Can you work these out from the model? Positions are in its coordinate system, mm. A direction names the side the tool comes from. Coordinates: 2 decimals unless noted, no trailing zeros. Loops run counter-clockwise (first coordinate to the right, second up) from the corner with the lowest first, then second, coordinate; pieces in that order, holes last. Notation, with made-up numbers: M 36.5,38.5 L 43.5,38.5 A29 ccw 43.5,67.5 Z; hole C -20.75,-12.5 d7. An arc over 180 degrees is marked long. Answer as a JSON object with one key per item and string values. Group by question number.
Item 1: We'd pull the mould along X, two halves only. Please class faces 3 (the cylindrical face through (16.345, -0.592, -0.479)), 4 (the flat face through (-4.945, -0.592, 35.75)), 5 (the flat face through (8.75, -0.59, -3.48)): +X half, -X half, draft (parallel to the pull), parting line (faces both ways), or undercut.
Item 2: Which directions (+Z, -Z, +X, -X, +Y, -Y) give clear straight access to the entire face, cutting with the end or side of a thin tool? Please do faces 1 (the flat face through (12.65, -0.59, 3.34)), 2 (the flat face through (5.34, -0.59, 15.32)).
Item 3: If I drill on line 1 (Z direction, x = -0.75, y = -0.8); line 2 (Z direction, x = 17.5, y = -0.5); line 3 (X direction, y = -0.5, z = 24), over which ranges is the centre line in solid material (lowest first)?
Item 4: Suppose I cut it at B-B (y = -0.5). Write out the boundary of the cut face in (x, z) (3 decimals).
Item 5: Suppose I cut it at C-C (x = 10.5). Write out the boundary of the cut face in (y, z).
Item 6: I'm going to push a flat-ended pin straight in: pin 1 Ø3 at (x, z) = (17.5, 0) entering from -Y. Where does the tip first touch, or does it pass through?
Item 7: Suppose I cut it at D-D (z = 6). Write out the boundary of the cut face in (x, y).
Item 8: Suppose I cut it at A-A (z = 39.38). Write out the boundary of the cut face in (x, y).
```python
from build123d import *

# Parameters (mm, degrees)
F0_R     = 1.6581186228
F1_DEPTH = 1.2


with BuildPart() as f1:
    # F0 (on Front) → F1 (new body)
    with BuildSketch(Plane.XZ):
        with BuildLine():
            ThreePointArc((1.25, 0), (-0.8838834765, -0.8838834765), (0, 1.25))
            Line((0, 1.25), (0, 3.8304899347))
            ThreePointArc((0, 3.8304899347), (-2.6634496965, 2.7529418545), (-3.8283991196, 0.126543752))
            Line((-3.8283991196, 0.126543752), (-3.7301566118, -0.8709677329))
            ThreePointArc((-3.7301566118, -0.8709677329), (-2.3198010798, -3.048143056), (0.1544652488, -3.8273742471))
            ThreePointArc((0.1544652488, -3.8273742471), (2.7626373921, -2.6533917501), (3.8304899347, 0))
            Line((3.8304899347, 0), (1.25, 0))
        make_face()
        with BuildLine():
            Line((0, 3.8304899347), (0, 1.25))
            ThreePointArc((0, 1.25), (0.8838834765, 0.8838834765), (1.25, 0))
            Line((1.25, 0), (3.8304899347, 0))
            ThreePointArc((3.8304899347, 0), (2.7085654081, 2.7085654081), (0, 3.8304899347))
        make_face()
        with BuildLine():
            ThreePointArc((-3.8283991196, 0.126543752), (-2.6634496965, 2.7529418545), (0, 3.8304899347))
            Line((0, 3.8304899347), (0, 18.75))
            ThreePointArc((0, 18.75), (-4.1368389571, 20.315017242), (-6.2019261398, 24.2262996982))
            Line((-6.2019261398, 24.2262996982), (-3.8283991196, 0.126543752))
        make_face()
        with BuildLine():
            Line((0, 18.75), (0, 3.8304899347))
            ThreePointArc((0, 3.8304899347), (2.7085654081, 2.7085654081), (3.8304899347, 0))
            Line((3.8304899347, 0), (14.375, 0))
            ThreePointArc((14.375, 0), (15.3390218203, 2.257387496), (17.6363109165, 3.122025678))
            Line((17.6363109165, 3.122025678), (7.5319273502, 3.5631936653))
            ThreePointArc((7.5319273502, 3.5631936653), (5.3080013875, 4.6346970575), (4.5523493544, 6.9847941218))
            Line((4.5523493544, 6.9847941218), (6.150289486, 23.8880471063))
            ThreePointArc((6.150289486, 23.8880471063), (4.0070434496, 20.2035322587), (0, 18.75))
        make_face()
        with BuildLine():
            Line((14.375, 0), (3.8304899347, 0))
            ThreePointArc((3.8304899347, 0), (2.7626373921, -2.6533917501), (0.1544652488, -3.8273742471))
            Line((0.1544652488, -3.8273742471), (17.5906089776, -3.1236861259))
            ThreePointArc((17.5906089776, -3.1236861259), (15.3225620623, -2.2415148957), (14.375, 0))
        make_face()
        with BuildLine():
            ThreePointArc((-6.2019261398, 24.2262996982), (-4.1368389571, 20.315017242), (0, 18.75))
            Line((0, 18.75), (0, 23.75))
            ThreePointArc((0, 23.75), (-1.25, 25), (0, 26.25))
            Line((0, 26.25), (0, 31.25))
            ThreePointArc((0, 31.25), (-4.1339767257, 29.6875085527), (-6.2009764026, 25.7812756582))
            ThreePointArc((-6.2009764026, 25.7812756582), (-6.2477972764, 25.1659192352), (-6.2337027111, 24.5489451152))
            Line((-6.2337027111, 24.5489451152), (-6.2019261398, 24.2262996982))
        make_face()
        with BuildLine():
            Line((0, 23.75), (0, 18.75))
            ThreePointArc((0, 18.75), (4.0070434496, 20.2035322587), (6.150289486, 23.8880471063))
            Line((6.150289486, 23.8880471063), (6.2497093523, 24.9397255246))
            Line((6.2497093523, 24.9397255246), (6.0440984205, 26.5910293157))
            ThreePointArc((6.0440984205, 26.5910293157), (3.8156629029, 29.9500723845), (0, 31.25))
            Line((0, 31.25), (0, 26.25))
            ThreePointArc((0, 26.25), (0.8838834765, 25.8838834765), (1.25, 25))
            ThreePointArc((1.25, 25), (0.8838834765, 24.1161165235), (0, 23.75))
        make_face()
        with BuildLine():
            Line((-3.7301566118, -0.8709677329), (-3.8283991196, 0.126543752))
            ThreePointArc((-3.8283991196, 0.126543752), (-3.8120464946, -0.375439294), (-3.7301566118, -0.8709677329))
        make_face()
        with BuildLine():
            ThreePointArc((17.6363109165, 3.122025678), (15.3390218203, 2.257387496), (14.375, 0))
            ThreePointArc((14.375, 0), (15.3225620623, -2.2415148957), (17.5906089776, -3.1236861259))
            ThreePointArc((17.5906089776, -3.1236861259), (19.7415148957, -2.1774379377), (20.625, 0))
            ThreePointArc((20.625, 0), (19.757387496, 2.1609781797), (17.6363109165, 3.122025678))
        make_face()
        with BuildLine():
            ThreePointArc((18.75, 0), (17.5, -1.25), (16.25, 0))
            ThreePointArc((16.25, 0), (17.5, 1.25), (18.75, 0))
        make_face(mode=Mode.SUBTRACT)
        with BuildLine():
            ThreePointArc((-6.2337027111, 24.5489451152), (-6.2199068518, 24.3874163287), (-6.2019261398, 24.2262996982))
            Line((-6.2019261398, 24.2262996982), (-6.2337027111, 24.5489451152))
        make_face()
        with BuildLine():
            Line((6.2497093523, 24.9397255246), (6.150289486, 23.8880471063))
            ThreePointArc((6.150289486, 23.8880471063), (6.222258406, 24.4117820738), (6.2497093523, 24.9397255246))
        make_face()
        with BuildLine():
            Line((6.0440984205, 26.5910293157), (6.2497093523, 24.9397255246))
            ThreePointArc((6.2497093523, 24.9397255246), (6.2499273376, 24.9698624119), (6.25, 25))
            ThreePointArc((6.25, 25), (6.1983108638, 25.8021486371), (6.0440984205, 26.5910293157))
        make_face()
        with BuildLine():
            ThreePointArc((-6.2009764026, 25.7812756582), (-4.1339767257, 29.6875085527), (0, 31.25))
            Line((0, 31.25), (0, 39.38))
            Line((0, 39.38), (0, 41.25))
            ThreePointArc((0, 41.25), (-2.8042828873, 42.5103218104), (-3.7236063691, 45.4441346731))
            Line((-3.7236063691, 45.4441346731), (-6.2009764026, 25.7812756582))
        make_face()
        with Locations((-1.9114875467, 39.38)):
            Circle(F0_R, mode=Mode.SUBTRACT)
        with BuildLine():
            Line((0, 39.38), (0, 31.25))
            ThreePointArc((0, 31.25), (3.8156629029, 29.9500723845), (6.0440984205, 26.5910293157))
            Line((6.0440984205, 26.5910293157), (3.7499672612, 45.015669719))
            ThreePointArc((3.7499672612, 45.015669719), (3.7499918153, 45.0078348766), (3.75, 45))
            ThreePointArc((3.75, 45), (2.6516504294, 42.3483495706), (0, 41.25))
            Line((0, 41.25), (0, 39.38))
        make_face()
        with BuildLine():
            ThreePointArc((3.7499672612, 45.015669719), (0.2146375512, 48.7438523905), (-3.7236063691, 45.4441346731))
            ThreePointArc((-3.7236063691, 45.4441346731), (-2.8042828873, 42.5103218104), (0, 41.25))
            ThreePointArc((0, 41.25), (2.6516504294, 42.3483495706), (3.75, 45))
            ThreePointArc((3.75, 45), (3.7499918153, 45.0078348766), (3.7499672612, 45.015669719))
        make_face()
        with BuildLine():
            ThreePointArc((1.25, 45), (0.8838834765, 44.1161165235), (0, 43.75))
            ThreePointArc((0, 43.75), (-0.8838834765, 45.8838834765), (1.25, 45))
        make_face(mode=Mode.SUBTRACT)
    extrude(amount=F1_DEPTH)


solid = f1.part
```
From the geometry:
{
 "1": {"face 3": "undercut", "face 4": "-X half", "face 5": "+X half"},
 "2": {"face 1": "+Z, +X, +Y, -Y", "face 2": "+X, +Y, -Y"},
 "3": {"line 1": "-3.76 to -1, 1 to 24, 26 to 38.2, 40.56 to 44, 46 to 48.67", "line 2": "-3.13 to -1.25, 1.25 to 3.13", "line 3": "-6.18 to -0.75, 0.75 to 6.17"},
 "4": {"outline": "M -6.202,24.226 L -3.828,0.127 A3.83 ccw 0.154,-3.827 L 17.591,-3.124 A3.125 ccw 17.636,3.122 L 7.532,3.563 A3.13 cw 4.552,6.985 L 6.15,23.888 A6.25 ccw 6.25,24.94 A6.25 ccw 6.25,25 A6.25 ccw 6.044,26.591 L 3.75,45.016 A3.75 ccw -3.724,45.444 L -6.201,25.781 A6.25 ccw Z; hole C -1.911,39.38 d3.316; hole C 0,0 d2.5; hole C 0,25 d2.5; hole C 0,45 d2.5; hole C 17.5,0 d2.5"},
 "5": {"outline": "M -1.2,-3.41 L 0,-3.41 L 0,3.43 L -1.2,3.43 Z"},
 "6": {"pin 1": "y = -1.2"},
 "7": {"outline": "M -4.41,-1.2 L 4.62,-1.2 L 4.62,0 L -4.41,0 Z"},
 "8": {"outline": "M -4.49,-1.2 L -3.57,-1.2 L -3.57,0 L -4.49,0 Z; M -0.25,-1.2 L 4.45,-1.2 L 4.45,0 L -0.25,0 Z"}
}
